Part print with two shaded views. Sizes in mm from the minimum x, y, z corner. A direction names the side the tool comes from. Give positions to 0.01 mm unless a question says otherwise; leave off trailing zeros. Write each loop counter-clockwise with the first axis right and the second up, starting at its lowest first coordinate (ties: lowest second). Pieces come first, ordered by that corner, then holes. Notation, with made-up numbers: (42.25, 87.5) -> (89.25, 87.5) arc R28 cw to (89.25, 123.5) -> close; hole circle Ø1 at (-26, 59.25). An arc over 180 degrees is marked (long way). Answer as a JSON object with one key per item and string values.
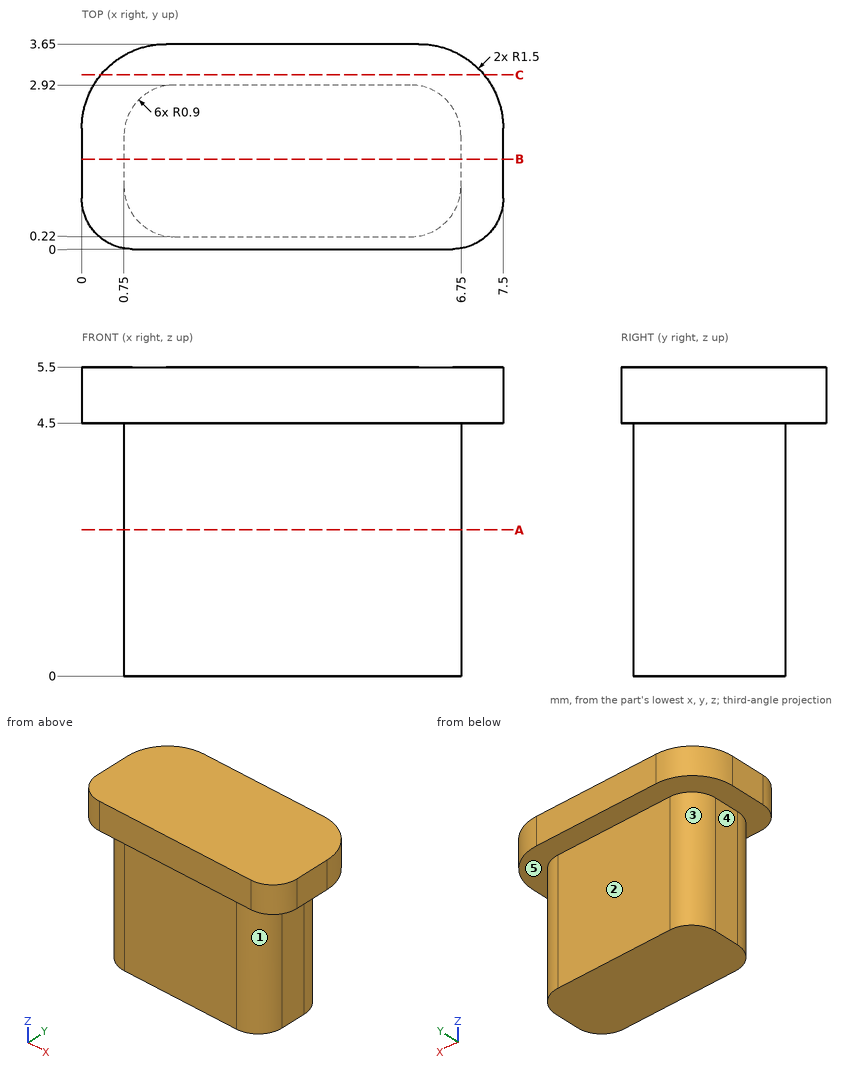
1) Slice it at B-B (y = 1.6). List the corners of the cut face in (x, z), then the cut area to 3 significant figures.
Model answer:
{"outline": "(0, 4.5) -> (0.75, 4.5) -> (0.75, 0) -> (6.75, 0) -> (6.75, 4.5) -> (7.5, 4.5) -> (7.5, 5.5) -> (0, 5.5) -> close", "area": "34.5 mm2"}
2) 3-axis set-ups, long thin cutter, end or side, ignore diameter. For the marked faces 1, 2, 3, 4 and 5: which of +Z, -Z, +X, -X, +Y, -Y reach the whole face in a straight line?
Model answer:
{"face 1": "-Z, +X, -Y", "face 2": "-Z, +X, -X, +Y", "face 3": "-Z, -X, +Y", "face 4": "-Z, -X, +Y, -Y", "face 5": "-Z"}
3) Slice it at A-A (z = 2.6). List the corners of the cut face in (x, y).
Model answer:
{"outline": "(0.75, 1.12) arc R0.9 ccw to (1.65, 0.22) -> (5.85, 0.22) arc R0.9 ccw to (6.75, 1.12) -> (6.75, 2.02) arc R0.9 ccw to (5.85, 2.92) -> (1.65, 2.92) arc R0.9 ccw to (0.75, 2.02) -> close"}
4) Slice it at C-C (y = 3.1). List the corners of the cut face in (x, z).
Model answer:
{"outline": "(0.34, 4.5) -> (7.16, 4.5) -> (7.16, 5.5) -> (0.34, 5.5) -> close"}
5) Pin check, flat tips, straight feed: pin 1 (1 mm diameter, centred on y = 1.5, z = 3.5, fed in from +X); pin 2 (1.3 mm diameter, centred on x = 3, z = 1.5, fed in from -Y); pin 3 (1.3 mm diameter, centred on x = 3.5, z = 1, fed in from +Y). Stop position of each tip, or through.
Model answer:
{"pin 1": "stops at x = 6.75", "pin 2": "stops at y = 0.22", "pin 3": "stops at y = 2.92"}
6) Wall check: probe 1 along Y at (x, z) = (2.75, 3.4); probe 2 along Z at (x, y) = (6.75, 3); probe 3 along X at (y, z) = (1.1, 3.75). Give the ranges that are in metal, low to high.
Model answer:
{"probe 1": "y = 0.22 to 2.92", "probe 2": "z = 4.5 to 5.5", "probe 3": "x = 0.75 to 6.75"}
